Geometry check sheet. Reference: the model listing, model coordinates, mm. A direction names the side the tool comes from. Give positions to 0.01 mm unless a question says otherwise; leave off trailing zeros. Write each loop counter-clockwise with the first axis right and the second up, starting at its lowest first coordinate (ties: lowest second). Pieces come first, ordered by that corner, then holes. Notation, with made-up numbers: (38.25, -31) - (42.25, -31) arc R19 ccw to (42.25, -6) - close; hole circle Ø11 at (-33.75, 76.5). An arc over 180 degrees is marked (long way). One line per question, with ' | ' between items. Start each with the question number.
Q1. Section check C-C on x = -13. Record the boundary of the cut face in (y, z).
Q2. Thickness scan on L1, parallel to Y at x = -26, z = 0.65; L2, parallel to Y at x = 0, z = 2.1; L3, parallel to X at y = -6.75, z = 1.45. Record the ranges inside material, lowest first. Write a range as [from, to].
Q3. Gauge pin test, flat ends, axial feed: P1, Ø8, axis at x = -6.533, y = -20.75, coming from the +Z side; P2, Ø1.7, axis at x = 0, y = 0, coming from the -Z side; P3, Ø4.5, axis at x = -49.5, y = -11.5, coming from the +Z side; P4, Ø12, axis at x = -26.5, y = -12.5, coming from the -Z side. Record the tip position at first contact, or that the pin passes through.
Q4. Section check A-A on x = -39. Record the boundary of the cut face in (y, z), and give its area (3 significant figures).
Q5. Section check B-B on y = -13.75. Record the boundary of the cut face in (x, z).
Q6. Set-up check for faces 5 (the face through (-50, -2, 4)), 6 (the face through (-25, 4, 1)), 7 (the face through (-0.4, -24.21, 1.59)), 8 (the face through (-9.236, -24.348, 1.594)), 9 (the face through (-31, -23.75, 1)): record each of +Z, -Z, +X, -X, +Y, -Y from which the full face is reachable in a straight line by a thin tool's end or side.
Q7. Release check for a two-part mould opening along X. For faces 1 (the face through (-25, -31, 1)), 2 (the face through (-0.45, -3.34, 1.59)), 3 (the face through (-52.128, -14, 1)), 4 (the face through (-47.984, -14, 1)) record: +X half, -X half, draft (parallel to the pull), parting line (faces both ways), or undercut.
```python
from build123d import *

# Parameters (mm, degrees)
EXTRUDE_1_DEPTH     = 1.2
SKETCH_2_8_R        = 1.5
EXTRUDE_7_DEPTH     = 2
SKETCH_2_9_R        = 2
SKETCH_2_9_R_2      = 1.5
EXTRUDE_8_DEPTH     = 5
SKETCH_2_10_R       = 2
SKETCH_2_10_R_2     = 1.5
EXTRUDE_9_DEPTH     = 5
SKETCH_2_11_R       = 2
SKETCH_2_11_R_2     = 1.5
EXTRUDE_10_DEPTH    = 5
SKETCH_2_12_R       = 2
SKETCH_2_12_R_2     = 1.5
EXTRUDE_11_DEPTH    = 5
SKETCH_2_13_R       = 1.5
SKETCH_2_13_R_2     = 0.75
EXTRUDE_12_DEPTH    = 5
SKETCH_2_14_R       = 1.5
SKETCH_2_14_R_2     = 0.75
EXTRUDE_13_DEPTH    = 5
SKETCH_2_15_R       = 1.5
SKETCH_2_15_R_2     = 0.75
EXTRUDE_14_DEPTH    = 5
SKETCH_2_16_R       = 1.5
SKETCH_2_16_R_2     = 0.75
EXTRUDE_15_DEPTH    = 5
SKETCH_2_19_R       = 1.5
SKETCH_2_19_R_2     = 0.75
CUT_EXTRUDE_4_DEPTH = 4
SKETCH_2_20_R       = 1.5
SKETCH_2_20_R_2     = 0.75
CUT_EXTRUDE_5_DEPTH = 4
SKETCH_2_21_R       = 1.5
SKETCH_2_21_R_2     = 0.75
CUT_EXTRUDE_6_DEPTH = 4
SKETCH_2_22_R       = 1.5
SKETCH_2_22_R_2     = 0.75
CUT_EXTRUDE_7_DEPTH = 4
EXTRUDE_16_DEPTH    = 3
EXTRUDE_18_DEPTH    = 2
EXTRUDE_19_DEPTH    = 1
SKETCH_5_W          = 0.85413001
SKETCH_5_H          = 2.598019217
SKETCH_5_W_2        = 1.005417368
SKETCH_5_H_2        = 2.475260341
CUT_EXTRUDE_9_DEPTH = 1


with BuildPart() as part:
    # Sketch 2 → Extrude 1 (new body)
    with BuildSketch(Plane.XY):
        with BuildLine():
            Line((-0.220057138, 2.999023685), (-49.204110666, 1.749023685))
            ThreePointArc((-49.204110666, 1.749023685), (-51.275787659, 0.844087888), (-52.127580054, -1.25))
            Line((-52.127580054, -1.25), (-52.127580054, -26.25))
            ThreePointArc((-52.127580054, -26.25), (-51.275787659, -28.344087888), (-49.204110666, -29.249023685))
            Line((-49.204110666, -29.249023685), (-0.220057138, -30.499023685))
            ThreePointArc((-0.220057138, -30.499023685), (2.04705122, -29.702759522), (3.007086332, -27.5))
            Line((3.007086332, -27.5), (3.007086332, 0))
            ThreePointArc((3.007086332, 0), (2.04705122, 2.202759522), (-0.220057138, 2.999023685))
        make_face()
        with BuildLine():
            ThreePointArc((2, -27.5), (0.750249731, -29.353948581), (-1.437125342, -28.890924423))
            Line((-1.437125342, -28.890924423), (-5.166627539, -25.037543154))
            ThreePointArc((-5.166627539, -25.037543154), (-9.188308261, -24.383089324), (-11.033, -20.75))
            Line((-11.033, -20.75), (-11.033, -6.75))
            ThreePointArc((-11.033, -6.75), (-9.188308261, -3.116910676), (-5.166627539, -2.462456846))
            Line((-5.166627539, -2.462456846), (-1.437125342, 1.390924423))
            ThreePointArc((-1.437125342, 1.390924423), (0.750249731, 1.853948581), (2, 0))
            ThreePointArc((2, 0), (1.853948581, -0.750249731), (1.437125342, -1.390924423))
            Line((1.437125342, -1.390924423), (-2.292376856, -5.244305693))
            ThreePointArc((-2.292376856, -5.244305693), (-2.098318267, -5.986064188), (-2.033, -6.75))
            Line((-2.033, -6.75), (-2.033, -20.75))
            ThreePointArc((-2.033, -20.75), (-2.098318267, -21.513935812), (-2.292376856, -22.255694307))
            Line((-2.292376856, -22.255694307), (1.437125342, -26.109075577))
            ThreePointArc((1.437125342, -26.109075577), (1.853948581, -26.749750269), (2, -27.5))
        make_face(mode=Mode.SUBTRACT)
        with BuildLine():
            ThreePointArc((-47.127580054, -26.25), (-49.127580054, -28.25), (-51.127580054, -26.25))
            Line((-51.127580054, -26.25), (-51.127580054, -1.25))
            ThreePointArc((-51.127580054, -1.25), (-49.127580054, 0.75), (-47.127580054, -1.25))
            Line((-47.127580054, -1.25), (-47.127580054, -3.75))
            Line((-47.127580054, -3.75), (-13.984053528, -3.75))
            Line((-13.984053528, -3.75), (-13.984053528, -13.75))
            Line((-13.984053528, -13.75), (-13.984053528, -23.75))
            Line((-13.984053528, -23.75), (-47.127580054, -23.75))
            Line((-47.127580054, -23.75), (-47.127580054, -26.25))
        make_face(mode=Mode.SUBTRACT)
    extrude(amount=EXTRUDE_1_DEPTH)

    # Sketch 2_8 → Extrude 7 (add)
    with BuildSketch(Plane.XY):
        with BuildLine():
            ThreePointArc((-11.033, -20.75), (-9.188308261, -24.383089324), (-5.166627539, -25.037543154))
            Line((-5.166627539, -25.037543154), (-6.415024561, -23.747679402))
            ThreePointArc((-6.415024561, -23.747679402), (-8.695628761, -18.670808609), (-3.533, -20.75))
            ThreePointArc((-3.533, -20.75), (-3.534944099, -20.857985255), (-3.540773877, -20.965830555))
            Line((-3.540773877, -20.965830555), (-2.292376856, -22.255694307))
            ThreePointArc((-2.292376856, -22.255694307), (-2.098318267, -21.513935812), (-2.033, -20.75))
            Line((-2.033, -20.75), (-2.033, -6.75))
            ThreePointArc((-2.033, -6.75), (-2.098318267, -5.986064188), (-2.292376856, -5.244305693))
            Line((-2.292376856, -5.244305693), (-3.540773877, -6.534169445))
            ThreePointArc((-3.540773877, -6.534169445), (-3.534944099, -6.642014745), (-3.533, -6.75))
            ThreePointArc((-3.533, -6.75), (-8.695628761, -8.829191391), (-6.415024561, -3.752320598))
            Line((-6.415024561, -3.752320598), (-5.166627539, -2.462456846))
            ThreePointArc((-5.166627539, -2.462456846), (-9.188308261, -3.116910676), (-11.033, -6.75))
            Line((-11.033, -6.75), (-11.033, -20.75))
        make_face()
        with Locations((-6.533, -13.75)):
            Circle(SKETCH_2_8_R, mode=Mode.SUBTRACT)
    extrude(amount=EXTRUDE_7_DEPTH)

    # Sketch 2_9 → Extrude 8 (add)
    with BuildSketch(Plane.XY):
        with Locations((-49.127580054, -1.25)):
            Circle(SKETCH_2_9_R)
        with Locations((-49.127580054, -1.25)):
            Circle(SKETCH_2_9_R_2, mode=Mode.SUBTRACT)
    extrude(amount=EXTRUDE_8_DEPTH)

    # Sketch 2_10 → Extrude 9 (add)
    with BuildSketch(Plane.XY):
        with Locations(Location((0, -27.5, 0), (0, 0, 224.064060962))):
            Circle(SKETCH_2_10_R)
        with Locations((0, -27.5)):
            Circle(SKETCH_2_10_R_2, mode=Mode.SUBTRACT)
    extrude(amount=EXTRUDE_9_DEPTH)

    # Sketch 2_11 → Extrude 10 (add)
    with BuildSketch(Plane.XY):
        with Locations(Location((0, 0, 0), (0, 0, 135.935939038))):
            Circle(SKETCH_2_11_R)
        Circle(SKETCH_2_11_R_2, mode=Mode.SUBTRACT)
    extrude(amount=EXTRUDE_10_DEPTH)

    # Sketch 2_12 → Extrude 11 (add)
    with BuildSketch(Plane.XY):
        with Locations((-49.127580054, -26.25)):
            Circle(SKETCH_2_12_R)
        with Locations((-49.127580054, -26.25)):
            Circle(SKETCH_2_12_R_2, mode=Mode.SUBTRACT)
    extrude(amount=EXTRUDE_11_DEPTH)

    # Sketch 2_13 → Extrude 12 (add)
    with BuildSketch(Plane.XY):
        with Locations((-49.127580054, -1.25)):
            Circle(SKETCH_2_13_R)
        with Locations((-49.127580054, -1.25)):
            Circle(SKETCH_2_13_R_2, mode=Mode.SUBTRACT)
    extrude(amount=EXTRUDE_12_DEPTH)

    # Sketch 2_14 → Extrude 13 (add)
    with BuildSketch(Plane.XY):
        with Locations((-49.127580054, -26.25)):
            Circle(SKETCH_2_14_R)
        with Locations((-49.127580054, -26.25)):
            Circle(SKETCH_2_14_R_2, mode=Mode.SUBTRACT)
    extrude(amount=EXTRUDE_13_DEPTH)

    # Sketch 2_15 → Extrude 14 (add)
    with BuildSketch(Plane.XY):
        Circle(SKETCH_2_15_R)
        Circle(SKETCH_2_15_R_2, mode=Mode.SUBTRACT)
    extrude(amount=EXTRUDE_14_DEPTH)

    # Sketch 2_16 → Extrude 15 (add)
    with BuildSketch(Plane.XY):
        with Locations((0, -27.5)):
            Circle(SKETCH_2_16_R)
        with Locations((0, -27.5)):
            Circle(SKETCH_2_16_R_2, mode=Mode.SUBTRACT)
    extrude(amount=EXTRUDE_15_DEPTH)

    # Sketch 2_19 → Cut-Extrude 4 (cut)
    with BuildSketch(Plane.XY):
        with Locations((-49.127580054, -1.25)):
            Circle(SKETCH_2_19_R)
        with Locations((-49.127580054, -1.25)):
            Circle(SKETCH_2_19_R_2, mode=Mode.SUBTRACT)
    extrude(amount=CUT_EXTRUDE_4_DEPTH, mode=Mode.SUBTRACT)

    # Sketch 2_20 → Cut-Extrude 5 (cut)
    with BuildSketch(Plane.XY):
        with Locations((-49.127580054, -26.25)):
            Circle(SKETCH_2_20_R)
        with Locations((-49.127580054, -26.25)):
            Circle(SKETCH_2_20_R_2, mode=Mode.SUBTRACT)
    extrude(amount=CUT_EXTRUDE_5_DEPTH, mode=Mode.SUBTRACT)

    # Sketch 2_21 → Cut-Extrude 6 (cut)
    with BuildSketch(Plane.XY):
        with Locations((0, -27.5)):
            Circle(SKETCH_2_21_R)
        with Locations((0, -27.5)):
            Circle(SKETCH_2_21_R_2, mode=Mode.SUBTRACT)
    extrude(amount=CUT_EXTRUDE_6_DEPTH, mode=Mode.SUBTRACT)

    # Sketch 2_22 → Cut-Extrude 7 (cut)
    with BuildSketch(Plane.XY):
        Circle(SKETCH_2_22_R)
        Circle(SKETCH_2_22_R_2, mode=Mode.SUBTRACT)
    extrude(amount=CUT_EXTRUDE_7_DEPTH, mode=Mode.SUBTRACT)

    # Sketch 2_23 → Extrude 16 (add)
    with BuildSketch(Plane.XY):
        with BuildLine():
            Line((-51.127580054, -1.25), (-51.127580054, -26.25))
            ThreePointArc((-51.127580054, -26.25), (-49.127580054, -24.25), (-47.127580054, -26.25))
            Line((-47.127580054, -26.25), (-47.127580054, -23.75))
            Line((-47.127580054, -23.75), (-47.984053528, -23.75))
            Line((-47.984053528, -23.75), (-47.984053528, -13.75))
            Line((-47.984053528, -13.75), (-47.984053528, -3.75))
            Line((-47.984053528, -3.75), (-47.127580054, -3.75))
            Line((-47.127580054, -3.75), (-47.127580054, -1.25))
            ThreePointArc((-47.127580054, -1.25), (-49.127580054, -3.25), (-51.127580054, -1.25))
        make_face()
    extrude(amount=EXTRUDE_16_DEPTH)

    # Sketch 2_24 → Extrude 18 (add)
    with BuildSketch(Plane.XY):
        with BuildLine():
            Line((-5.166627539, -25.037543154), (-1.437125342, -28.890924423))
            ThreePointArc((-1.437125342, -28.890924423), (-1.390924423, -26.062874658), (1.437125342, -26.109075577))
            Line((1.437125342, -26.109075577), (-2.292376856, -22.255694307))
            ThreePointArc((-2.292376856, -22.255694307), (-3.403420047, -23.983532019), (-5.166627539, -25.037543154))
        make_face()
        with BuildLine():
            Line((-6.415024561, -23.747679402), (-5.166627539, -25.037543154))
            ThreePointArc((-5.166627539, -25.037543154), (-3.403420047, -23.983532019), (-2.292376856, -22.255694307))
            Line((-2.292376856, -22.255694307), (-3.540773877, -20.965830555))
            ThreePointArc((-3.540773877, -20.965830555), (-4.446613365, -22.905688013), (-6.415024561, -23.747679402))
        make_face()
        with BuildLine():
            ThreePointArc((-2.292376856, -5.244305693), (-3.403420047, -3.516467981), (-5.166627539, -2.462456846))
            Line((-5.166627539, -2.462456846), (-6.415024561, -3.752320598))
            ThreePointArc((-6.415024561, -3.752320598), (-4.446613365, -4.594311987), (-3.540773877, -6.534169445))
            Line((-3.540773877, -6.534169445), (-2.292376856, -5.244305693))
        make_face()
        with BuildLine():
            Line((-1.437125342, 1.390924423), (-5.166627539, -2.462456846))
            ThreePointArc((-5.166627539, -2.462456846), (-3.403420047, -3.516467981), (-2.292376856, -5.244305693))
            Line((-2.292376856, -5.244305693), (1.437125342, -1.390924423))
            ThreePointArc((1.437125342, -1.390924423), (-1.390924423, -1.437125342), (-1.437125342, 1.390924423))
        make_face()
    extrude(amount=EXTRUDE_18_DEPTH)

    # Sketch 4 → Extrude 19 (add)
    with BuildSketch(Plane(origin=(0, 0, 0), x_dir=(-1, 0, 0), z_dir=(0, 0, -1))):
        with BuildLine():
            Line((27.712083902, 2.374023685), (27.712083902, -0.625976315))
            ThreePointArc((27.712083902, -0.625976315), (24.712083902, -3.625976315), (21.712083902, -0.625976315))
            Line((21.712083902, -0.625976315), (21.712083902, 2.374023685))
            ThreePointArc((21.712083902, 2.374023685), (24.712083902, 5.374023685), (27.712083902, 2.374023685))
        make_face()
        with BuildLine():
            Line((21.712083902, -29.874023685), (21.712083902, -26.874023685))
            ThreePointArc((21.712083902, -26.874023685), (24.712083902, -23.874023685), (27.712083902, -26.874023685))
            Line((27.712083902, -26.874023685), (27.712083902, -29.874023685))
            ThreePointArc((27.712083902, -29.874023685), (24.712083902, -32.874023685), (21.712083902, -29.874023685))
        make_face()
    extrude(amount=-EXTRUDE_19_DEPTH)

    # Sketch 5 → Cut-Extrude 9 (cut)
    with BuildSketch(Plane.XY.offset(1)):
        with Locations((-25.795795215, -29.846368989)):
            Rectangle(SKETCH_5_W, SKETCH_5_H)
        with Locations((-23.726763116, -29.899167603)):
            Rectangle(SKETCH_5_W_2, SKETCH_5_H_2)
    extrude(amount=-CUT_EXTRUDE_9_DEPTH, mode=Mode.SUBTRACT)


solid = part.part
```
Working result:
1) outline: (-30.17, 0) - (2.67, 0) - (2.67, 1.2) - (-30.17, 1.2) - close
2) L1: y = [-32.58, -31.15], [-28.55, -23.75], [-3.75, 5.08] | L2: y = [-29.5, -29], [-26, -25.5], [-2, -1.5], [1.5, 2] | L3: x = [-51.13, -47.98], [-11.03, -9.53], [-3.53, -2.03]
3) P1: stops at z = 2 | P2: stops at z = 4 | P3: stops at z = 3 | P4: passes through
4) outline: (-29.51, 0) - (-23.75, 0) - (-23.75, 1.2) - (-29.51, 1.2) - close; (-3.75, 0) - (2.01, 0) - (2.01, 1.2) - (-3.75, 1.2) - close | area: 13.8 mm2
5) outline: (-52.13, 0) - (-47.98, 0) - (-47.98, 3) - (-51.13, 3) - (-51.13, 1.2) - (-52.13, 1.2) - close; (-13.98, 0) - (-8.03, 0) - (-8.03, 2) - (-11.03, 2) - (-11.03, 1.2) - (-13.98, 1.2) - close; (-5.03, 0) - (3.01, 0) - (3.01, 1.2) - (-2.03, 1.2) - (-2.03, 2) - (-5.03, 2) - close
6) face 5: -Z | face 6: +Z, -X, +Y | face 7: +Z, +X | face 8: +Z, -Y | face 9: +Z, -Z
7) face 1: draft | face 2: +X half | face 3: -X half | face 4: undercut
